```python
from build123d import *

# Parameters (mm, degrees)
SKETCH1_W           = 19.05
SKETCH1_H           = 57.15
BOSS_EXTRUDE1_DEPTH = 19.05
SKETCH2_W           = 12.7
SKETCH2_H           = 12.7
CUT_EXTRUDE1_DEPTH  = 76.2
SKETCH3_W           = 2.54
SKETCH3_H           = 5.08
BOSS_EXTRUDE2_DEPTH = 2.54
SKETCH4_R           = 0.508
SKETCH4_R_2         = 1.5875
CUT_EXTRUDE2_DEPTH  = 19.05
SKETCH7_R           = 0.508
CUT_EXTRUDE3_DEPTH  = 12.7
SKETCH8_W           = 12.7
SKETCH8_H           = 9.525
CUT_EXTRUDE4_DEPTH  = 25.4
SKETCH11_R          = 1.5875
CUT_EXTRUDE6_DEPTH  = 19.05
SKETCH12_W          = 12.7
SKETCH12_H          = 30.970960978
CUT_EXTRUDE7_DEPTH  = 3.81
SKETCH13_W          = 12.7
SKETCH13_H          = 19.463069007
CUT_EXTRUDE8_DEPTH  = 3.81
CUT_EXTRUDE9_DEPTH  = 19.05


with BuildPart() as part:
    # Sketch1 → Boss-Extrude1 (new body)
    with BuildSketch(Plane(origin=(0, 0, 0), x_dir=(1, 0, 0), z_dir=(0, 1, 0))):
        with Locations((9.525, 28.575)):
            Rectangle(SKETCH1_W, SKETCH1_H)
    extrude(amount=BOSS_EXTRUDE1_DEPTH)

    # Sketch2 → Cut-Extrude1 (cut)
    with BuildSketch(Plane.XY):
        with Locations((9.525, 9.525)):
            Rectangle(SKETCH2_W, SKETCH2_H)
    extrude(amount=-CUT_EXTRUDE1_DEPTH, mode=Mode.SUBTRACT)

    # Sketch3 → Boss-Extrude2 (add)
    with BuildSketch(Plane(origin=(0, 19.05, 0), x_dir=(1, 0, 0), z_dir=(0, 1, 0))):
        with Locations((8.89, 24.13)):
            Rectangle(SKETCH3_W, SKETCH3_H)
    extrude(amount=BOSS_EXTRUDE2_DEPTH)

    # Sketch4 → Cut-Extrude2 (cut)
    with BuildSketch(Plane(origin=(0, 0, 0), x_dir=(0, 0, -1), z_dir=(1, 0, 0))):
        with Locations((24.13, 20.32)):
            Circle(SKETCH4_R)
        with Locations((9.525, 9.525)):
            Circle(SKETCH4_R_2)
        with BuildLine():
            ThreePointArc((26.67, 19.05), (24.13, 24.78976855), (21.59, 19.05))
            add(Edge.make_bspline(
                [(26.67, 19.05), (26.67, 21.59), (24.13, 21.59), (21.59, 21.59), (21.59, 19.05)],
                knots=[3.141592654, 3.141592654, 3.141592654, 4.71238898, 4.71238898, 6.283185307, 6.283185307, 6.283185307], degree=2, weights=[1, 0.707106781, 1, 0.707106781, 1]))
        make_face()
        with BuildLine():
            ThreePointArc((9.525, 19.05), (0, 9.525), (9.525, 0))
            ThreePointArc((9.525, 0), (-29.420443119, 9.525), (9.525, 19.05))
        make_face()
    extrude(amount=CUT_EXTRUDE2_DEPTH, mode=Mode.SUBTRACT)

    # Sketch7 → Cut-Extrude3 (cut)
    with BuildSketch(Plane(origin=(0, 19.05, 0), x_dir=(1, 0, 0), z_dir=(0, 1, 0))):
        with Locations((9.525, 36.83)):
            Circle(SKETCH7_R)
        Polygon((3.175, 0), (3.175, 11.43), (6.35, 11.43), (12.7, 11.43), (15.875, 11.43), (15.875, 0), align=None)
    extrude(amount=-CUT_EXTRUDE3_DEPTH, mode=Mode.SUBTRACT)

    # Sketch8 → Cut-Extrude4 (cut)
    with BuildSketch(Plane(origin=(0, 19.05, 0), x_dir=(1, 0, 0), z_dir=(0, 1, 0))):
        with Locations((9.525, 4.7625)):
            Rectangle(SKETCH8_W, SKETCH8_H)
    extrude(amount=-CUT_EXTRUDE4_DEPTH, mode=Mode.SUBTRACT)

    # Sketch11 → Cut-Extrude6 (cut)
    with BuildSketch(Plane(origin=(0, 0, 0), x_dir=(0, 0, -1), z_dir=(1, 0, 0))):
        with Locations((47.625, 9.525)):
            Circle(SKETCH11_R)
        with BuildLine():
            ThreePointArc((47.625, 0), (57.15, 9.525), (47.625, 19.05))
            ThreePointArc((47.625, 19.05), (63.905355935, 9.525), (47.625, 0))
        make_face()
    extrude(amount=CUT_EXTRUDE6_DEPTH, mode=Mode.SUBTRACT)

    # Sketch12 → Cut-Extrude7 (cut)
    with BuildSketch(Plane(origin=(0, 19.05, 0), x_dir=(1, 0, 0), z_dir=(0, 1, 0))):
        with Locations((9.525, 53.585480489)):
            Rectangle(SKETCH12_W, SKETCH12_H)
    extrude(amount=-CUT_EXTRUDE7_DEPTH, mode=Mode.SUBTRACT)

    # Sketch13 → Cut-Extrude8 (cut)
    with BuildSketch(Plane(origin=(0, 0, 0), x_dir=(1, 0, 0), z_dir=(0, 1, 0))):
        with Locations((9.525, 57.356534504)):
            Rectangle(SKETCH13_W, SKETCH13_H)
    extrude(amount=CUT_EXTRUDE8_DEPTH, mode=Mode.SUBTRACT)

    # Sketch14 → Cut-Extrude9 (cut)
    with BuildSketch(Plane(origin=(0, 0, 0), x_dir=(0, 0, -1), z_dir=(1, 0, 0))):
        with BuildLine():
            Line((9.525, 0), (9.525, 3.175))
            ThreePointArc((9.525, 3.175), (5.21507822, 5.21507822), (3.175, 9.525))
            Line((3.175, 9.525), (3.175, 18.741336737))
            Line((3.175, 18.741336737), (-3.728591213, 9.978700773))
            Line((-3.728591213, 9.978700773), (-2.544461104, 0))
            Line((-2.544461104, 0), (9.525, 0))
        make_face()
        with BuildLine():
            Line((47.625, 0), (47.625, 3.175))
            ThreePointArc((47.625, 3.175), (52.115128061, 5.034871939), (53.975, 9.525))
            Line((53.975, 9.525), (53.975, 20.201145039))
            Line((53.975, 20.201145039), (59.422737854, 9.525))
            Line((59.422737854, 9.525), (58.062916797, -0.332636104))
            Line((58.062916797, -0.332636104), (47.625, 0))
        make_face()
    extrude(amount=CUT_EXTRUDE9_DEPTH, mode=Mode.SUBTRACT)


solid = part.part
```
The model under review builds one solid part; all positions refer to its coordinate system, in mm. A direction names the side the tool comes from. Round coordinates to 2 decimals unless told otherwise and drop trailing zeros. Write each loop counter-clockwise with the first axis right and the second up, starting at its lowest first coordinate (ties: lowest second). Pieces come first, ordered by that corner, then holes.
(1) We need section C-C on z = -42. Give the boundary of the cut face in (x, y) (3 decimals).
(2) We need section A-A on x = 5. Give the boundary of the cut face in (y, z) (3 decimals), and give its area (3 significant figures).
(3) Mouldability with a two-part tool opening along Y and no side actions: class faces 1 (the flat face through (3.175, 11, -28)), 2 (the flat face through (17, 13, -3.175)), 3 (the flat face through (9, 0, -29)) as +Y half, -Y half, draft (parallel to the pull), parting line (faces both ways), or undercut.
(4) Insertion check: pin 1 (2 mm diameter, centred on y = 20.5, z = -24.5, fed in from -X); pin 2 (3 mm diameter, centred on x = 10, y = 16.5, fed in from -Z); pin 3 (8 mm diameter, centred on x = 6, z = -36, fed in from +Y); pin 4 (5 mm diameter, centred on x = 14, y = 18, fed in from -Z) (3 decimals). Each pin has a flat end and moves straight along its axis. Give the tip position at first contact, or say it passes through.
(5) We need section B-B on y = 13. Give the boundary of the cut face in (x, z) (3 decimals).
(6) Machinability: for faces 4 (the cylindrical face through (17.44, 18.406, -51.069)), 5 (the flat face through (9, 15.875, -25)), 6 (the flat face through (9, 2, -47.625)), which of the approach directions +Z, -Z, +X, -X, +Y, -Y give a long, thin tool a straight path to every point of the face, cutting with its end or side? Answer none if there is none.
(7) Wall thickness on L1, parallel to Y at x = 3.75, z = -30 (3 decimals); L2, parallel to X at y = 18.05, z = -36.83: over which ranges is each line inside the solid? List them lowest first.
(8) We need section D-D on x = 2. Give the number of separate pieces and of enclosed holes in the cut face, and give its area (3 significant figures).
Findings below:
1. outline: (0, 0) - (19.05, 0) - (19.05, 19.05) - (15.875, 19.05) - (15.875, 3.175) - (3.175, 3.175) - (3.175, 19.05) - (0, 19.05) - close
2. outline: (0, -47.625) - (3.175, -47.625) - (3.175, -9.525) - (0, -9.525) - close; (15.875, -38.1) - (19.05, -38.1) - (19.05, -11.43) - (15.875, -11.43) - close
2. area: 206 mm2
3. face 1: undercut
3. face 2: draft
3. face 3: -Y half
4. pin 1: stops at x = 7.62
4. pin 2: stops at z = -38.1
4. pin 3: stops at y = 19.05
4. pin 4: stops at z = -53.975
5. outline: (0, -53.975) - (3.175, -53.975) - (3.175, -3.175) - (0, -3.175) - close; (15.875, -53.975) - (19.05, -53.975) - (19.05, -3.175) - (15.875, -3.175) - close
6. face 4: -Z, +X, -X, +Y
6. face 5: +Z, -Z
6. face 6: -Z, +X, -X, -Y
7. L1: y = 0 to 3.175, 15.875 to 19.05
7. L2: x = 0 to 9.02, 10.03 to 19.05
8. separate pieces: 1
8. enclosed holes: 2
8. area: 883 mm2
